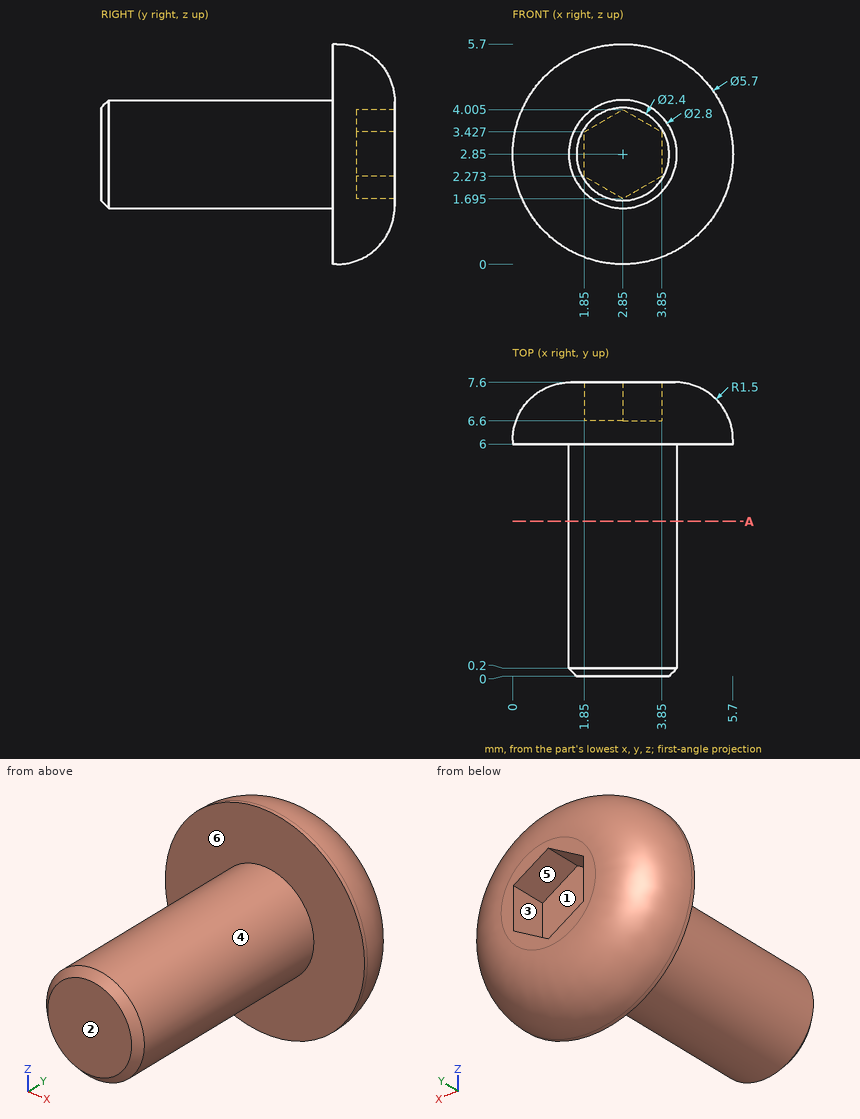
Input: dimensioned drawing with shaded views. Units: mm. Origin: part minimum x, y, z. A direction names the side the tool comes from. Round coordinates to 2 decimals unless told otherwise and drop trailing zeros. Loops run counter-clockwise (first coordinate to the right, second up) from the corner with the lowest first, then second, coordinate; pieces in that order, holes last. Notation, with made-up numbers: (34, -38.75) -> (93, -38.75) arc R18 cw to (93, -4.75) -> close; hole circle Ø7 at (15, -30.75). An arc over 180 degrees is marked (long way). Answer as a JSON object with one key per item and string values. Group by question number.
Q1. Contact query for flat-ended pins moving along their axis: P1, Ø1.5, axis at y = 1, z = 4.5, coming from the +X side; P2, Ø2, axis at y = 4.5, z = 2, coming from the -X side; P3, Ø3, axis at x = 4.5, y = 5.5, coming from the +Z side. Output: stop coordinate, or through.
Q2. Ray query, line 1 (Y direction, x = 3.2, z = 2.2); line 2 (Z direction, x = 5.35, y = 6.25) (1 decimal); line 3 (Z direction, x = 4.05, y = 7). Return the intervals inside material, ascending. Write a range as from..to.
Q3. Mould query, pull axis X, two halves, no side actions, for the marked faces 1, 2, 3 and 4. Classes: pulls with the +X half, pulls with the -X half, needs draft (parallel to the pull), parting line crosses it, or undercut.
Q4. Access query for the marked faces 5 and 6. Directions: +Z, -Z, +X, -X, +Y, -Y. A direction counts if a zero-diameter tool reaches every point of the face in a straight line with its end or side. Return the directions, or none.
Q5. Section query A-A (y = 4). Output: boundary loops of the cut face in (x, z).
Completed:
{
 "1": {"P1": "x = 3.92", "P2": "x = 1.45", "P3": "z = 5.69"},
 "2": {"line 1": "0..6.6", "line 2": "1.5..4.2", "line 3": "0.6..5.1"},
 "3": {"face 1": "undercut", "face 2": "needs draft", "face 3": "undercut", "face 4": "parting line crosses it"},
 "4": {"face 5": "+Y", "face 6": "-Y"},
 "5": {"outline": "circle Ø2.8 at (2.85, 2.85)"}
}
